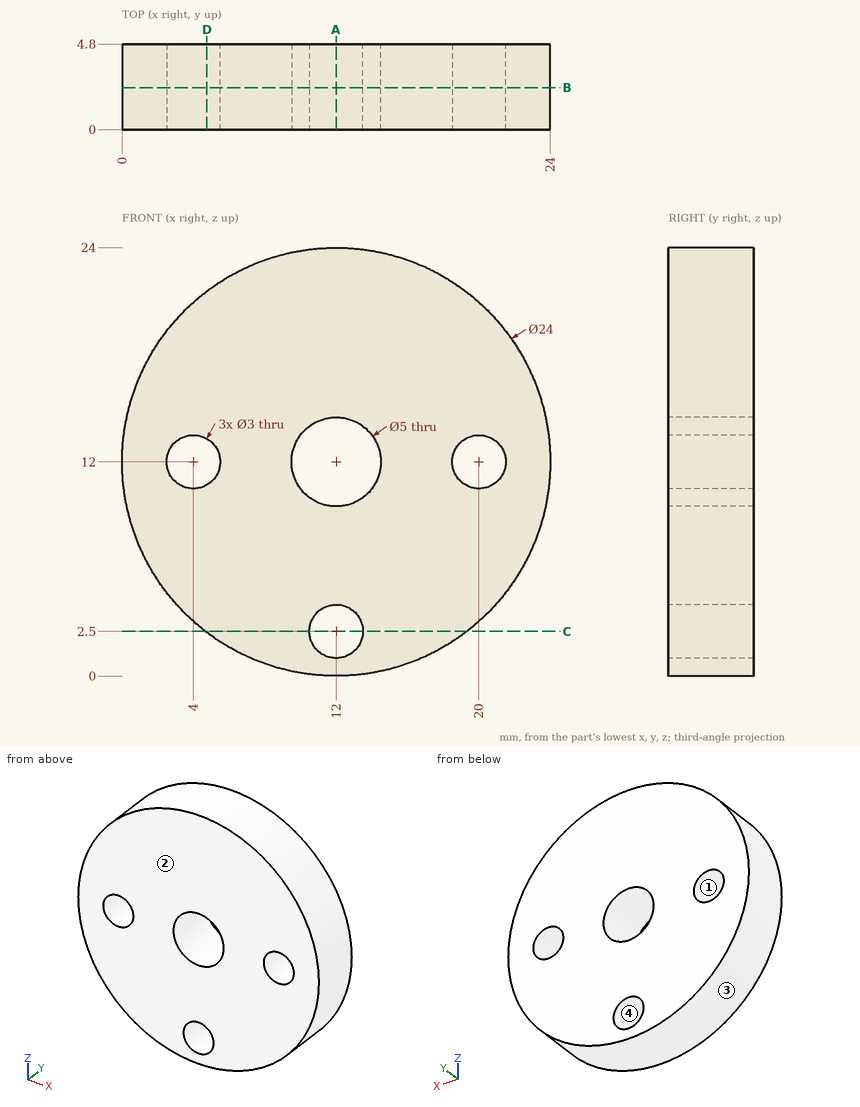
For this review, use the dimensioned drawing (mm, ordinates from the lowest corner) and the shaded views. Round coordinates to 2 decimals unless told otherwise and drop trailing zeros. Write each loop counter-clockwise with the first axis right and the second up, starting at its lowest first coordinate (ties: lowest second). Pieces come first, ordered by that corner, then holes. Notation, with made-up numbers: (-2, -5.75) - (42, -5.75) arc R14 ccw to (42, 1.25) - close; hole circle Ø1 at (-26.5, -14.75). An arc over 180 degrees is marked (long way). Answer as a JSON object with one key per item and string values.
1. We need section D-D on x = 4.75. Give the boundary of the cut face in (y, z).
Response values:
{"outline": "(0, 2.44) - (4.8, 2.44) - (4.8, 10.7) - (0, 10.7) - close; (0, 13.3) - (4.8, 13.3) - (4.8, 21.56) - (0, 21.56) - close"}
2. We need section A-A on x = 12. Give the boundary of the cut face in (y, z), then the cut area to 3 significant figures.
Response values:
{"outline": "(0, 0) - (4.8, 0) - (4.8, 1) - (0, 1) - close; (0, 4) - (4.8, 4) - (4.8, 9.5) - (0, 9.5) - close; (0, 14.5) - (4.8, 14.5) - (4.8, 24) - (0, 24) - close", "area": "76.8 mm2"}
3. Draft analysis for pull direction Z (two halves, no side actions). For the marked faces 1, 2, 3 and 4, state which applies: +Z half, -Z half, draft (parallel to the pull), parting line (faces both ways), or undercut.
Response values:
{"face 1": "undercut", "face 2": "draft", "face 3": "parting line", "face 4": "undercut"}
4. We need section C-C on z = 2.5. Give the boundary of the cut face in (x, y).
Response values:
{"outline": "(4.67, 0) - (10.5, 0) - (10.5, 4.8) - (4.67, 4.8) - close; (13.5, 0) - (19.33, 0) - (19.33, 4.8) - (13.5, 4.8) - close"}
5. For pin 1 Ø5 at (x, z) = (12, 2.5) entering from -Y; pin 2 Ø1.5 at (x, y) = (7.5, 1) entering from +Z; pin 3 Ø1 at (y, z) = (3.5, 9.5) entering from +X; pin 4 Ø4 at (x, z) = (12, 12) entering from -Y, all flat-tipped, find the tip position at first contact; note any pin that passes through.
Response values:
{"pin 1": "stops at y = 0", "pin 2": "stops at z = 23.4", "pin 3": "stops at x = 23.83", "pin 4": "passes through"}
6. To check wall thickness, follow line 1 along Z through (x, y) = (12, 1.85); line 2 along X through (y, z) = (1.4, 12); line 3 along X through (y, z) = (0.7, 13). State the ranges of each line that lie inside material, in increasing order.
Response values:
{"line 1": "z = 0 to 1, 4 to 9.5, 14.5 to 24", "line 2": "x = 0 to 2.5, 5.5 to 9.5, 14.5 to 18.5, 21.5 to 24", "line 3": "x = 0.04 to 2.88, 5.12 to 9.71, 14.29 to 18.88, 21.12 to 23.96"}
7. We need section B-B on y = 2.35. Give the boundary of the cut face in (x, z).
Response values:
{"outline": "circle Ø24 at (12, 12); hole circle Ø3 at (4, 12); hole circle Ø5 at (12, 12); hole circle Ø3 at (12, 2.5); hole circle Ø3 at (20, 12)"}
